```python
from build123d import *

# Parameters (mm, degrees)
SKETCH1_W           = 139.7
SKETCH1_H           = 203.2
BOSS_EXTRUDE1_DEPTH = 3.18
SKETCH2_R           = 1.5
SKETCH2_W           = 3.18
SKETCH2_H           = 91.725
CUT_EXTRUDE1_DEPTH  = 124.335700022
SKETCH3_R           = 8.441994665
CUT_EXTRUDE2_DEPTH  = 10
SKETCH5_W           = 25.530623926
SKETCH5_H           = 65.176444071
CUT_EXTRUDE3_DEPTH  = 10


with BuildPart() as part:
    # Sketch1 → Boss-Extrude1 (new body)
    with BuildSketch(Plane.XY):
        Rectangle(SKETCH1_W, SKETCH1_H)
    extrude(amount=BOSS_EXTRUDE1_DEPTH)

    # Sketch2 → Cut-Extrude1 (cut, through all)
    with BuildSketch(Plane.XY.offset(3.18)):
        with Locations((-67.85, 0)):
            Circle(SKETCH2_R)
        with Locations((67.85, 0)):
            Circle(SKETCH2_R)
        Polygon((-10, 101.6), (10, 101.6), (10, 98.42), (1.5, 98.42), (1.5, 94.42), (3.5, 94.42), (3.5, 91.42), (1.5, 91.42), (1.5, 88.42), (-1.5, 88.42), (-1.5, 91.42), (-3.5, 91.42), (-3.5, 94.42), (-1.5, 94.42), (-1.5, 98.42), (-10, 98.42), align=None)
        Polygon((-10, -101.6), (-10, -98.42), (-1.5, -98.42), (-1.5, -94.42), (-3.5, -94.42), (-3.5, -91.42), (-1.5, -91.42), (-1.5, -88.42), (1.5, -88.42), (1.5, -91.42), (3.5, -91.42), (3.5, -94.42), (1.5, -94.42), (1.5, -98.42), (10, -98.42), (10, -101.6), align=None)
        with Locations((-68.26, 55.7375)):
            Rectangle(SKETCH2_W, SKETCH2_H)
        with Locations((-68.26, -55.7375)):
            Rectangle(SKETCH2_W, SKETCH2_H)
        with Locations((68.26, -55.7375)):
            Rectangle(SKETCH2_W, SKETCH2_H)
        with Locations((68.26, 55.7375)):
            Rectangle(SKETCH2_W, SKETCH2_H)
    extrude(amount=-CUT_EXTRUDE1_DEPTH, mode=Mode.SUBTRACT)

    # Sketch3 → Cut-Extrude2 (cut)
    with BuildSketch(Plane(origin=(0, 0, 0), x_dir=(-1, 0, 0), z_dir=(0, 0, -1))):
        with Locations((0.068813102, -81.648638462)):
            Circle(SKETCH3_R)
    extrude(amount=-CUT_EXTRUDE2_DEPTH, mode=Mode.SUBTRACT)

    # Sketch5 → Cut-Extrude3 (cut)
    with BuildSketch(Plane(origin=(0, 0, 0), x_dir=(-1, 0, 0), z_dir=(0, 0, -1))):
        with Locations((0, 52.074409839)):
            Rectangle(SKETCH5_W, SKETCH5_H)
    extrude(amount=-CUT_EXTRUDE3_DEPTH, mode=Mode.SUBTRACT)


solid = part.part
```
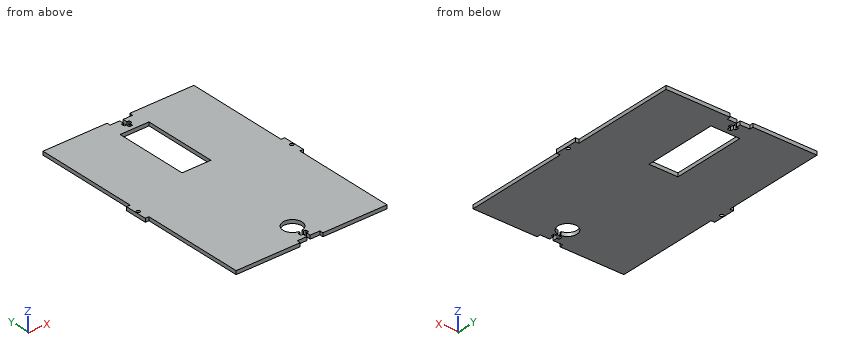
Input: part model. Units: mm. Frame: model coordinates. Give positions to 0.01 mm unless a question says otherwise; leave off trailing zeros. Order: outer loops, then holes, each group sorted by start corner. A loop starts at its lowest first (then second) coordinate and runs counter-clockwise, first axis right, second up. Notation, with made-up numbers: M -34.5,1.5 L -26.5,1.5 A16 cw -26.5,10.5 Z; hole C 8,45.5 d6. An arc over 180 degrees is marked long. Return JSON: item names as keys, results as strings.
1) Contact query for flat-ended pins moving along their axis: pin 1 (1 mm diameter, centred on x = -2.5, z = 2, fed in from -Y); pin 2 (1.5 mm diameter, centred on y = -39.5, z = 2, fed in from -X); pin 3 (1 mm diameter, centred on x = 3, z = 1.5, fed in from +Y). Output: stop coordinate, or through.
Taken from the geometry:
{"pin 1": "stops at y = -98.42", "pin 2": "stops at x = -66.67", "pin 3": "stops at y = 98.42"}
2) Section query D-D on y = -15.5. Output: boundary loops of the cut face in (x, z), and give its area (3 significant figures).
Taken from the geometry:
{"outline": "M -66.67,0 L 66.67,0 L 66.67,3.18 L -66.67,3.18 Z", "area": "424 mm2"}
3) Section query C-C on z = 2.15. Count the separate pieces of the cut face and the enclosed holes in it, and give its area (3 significant figures).
Taken from the geometry:
{"separate pieces": "1", "enclosed holes": "3", "area": "25,100 mm2"}
4) Section query A-A on y = 46. Output: boundary loops of the cut face in (x, z), and give its area (3 significant figures).
Taken from the geometry:
{"outline": "M -66.67,0 L -12.77,0 L -12.77,3.18 L -66.67,3.18 Z; M 12.77,0 L 66.67,0 L 66.67,3.18 L 12.77,3.18 Z", "area": "343 mm2"}
5) Section query B-B on y = -86. Output: boundary loops of the cut face in (x, z).
Taken from the geometry:
{"outline": "M -66.67,0 L -7.3,0 L -7.3,3.18 L -66.67,3.18 Z; M 7.17,0 L 66.67,0 L 66.67,3.18 L 7.17,3.18 Z"}
6) Line query: L1, parallel to Y at x = -67.85, z = 1.15 (3 decimals); L2, parallel to Y at x = 6, z = 1.4; L3, parallel to X at y = 33, z = 0.75. Output: solid intervals per line, ascending. Write a range as [from, to].
Taken from the geometry:
{"L1": "y = [-9.875, -1.5], [1.5, 9.875]", "L2": "y = [-98.42, -87.52], [-75.78, 19.49], [84.66, 98.42]", "L3": "x = [-66.67, -12.77], [12.77, 66.67]"}
